```python
from build123d import *

# Parameters (mm, degrees)
F0_R     = 5
F1_DEPTH = 3


with BuildPart() as f1:
    # F0 (on Right) → F1 (new body)
    with BuildSketch(Plane.YZ):
        with BuildLine():
            ThreePointArc((30, 15), (15.633379, 6.233241), (0, 0))
            Line((0, 0), (30, 0))
            Line((30, 0), (30, -23))
            ThreePointArc((30, -23), (37.5, -30.5), (45, -23))
            Line((45, -23), (45, 6.824179))
            ThreePointArc((45, 6.824179), (43.227486, 10.642992), (39.166667, 11.754245))
            ThreePointArc((39.166667, 11.754245), (34.162235, 12.187856), (30, 15))
        make_face()
        with Locations((37.5, -23)):
            Circle(F0_R, mode=Mode.SUBTRACT)
    extrude(amount=F1_DEPTH)


solid = f1.part
```
The listing builds one solid part. Answer for the finished solid, in the listing's coordinates (mm). A direction names the side the tool comes from. Round coordinates to 2 decimals unless told otherwise and drop trailing zeros. Loops run counter-clockwise (first coordinate to the right, second up) from the corner with the lowest first, then second, coordinate; pieces in that order, holes last. Notation, with made-up numbers: (32.25, -6.5) - (47.25, -6.5) arc R15 cw to (47.25, 11.5) - close; hole circle Ø4 at (3, 14.25). An arc over 180 degrees is marked (long way). Use one line per item in the form item = value. Start each with the question number.
1. A tool of negligible diameter and unlimited length cuts with its end or side. For faces 1 (the face through (3, 32, -3)), 2 (the face through (1, 30, -11)), from which of +Z, -Z, +X, -X, +Y, -Y can it reach the whole face along a straight path? Write none if from no direction.
2. The part is cut by section C-C on z = -15. Determine the outline of the cut face in (x, y), then the cut area to 3 significant figures.
3. The part is cut by section A-A on y = 37.5. Determine the outline of the cut face in (x, z), then the cut area to 3 significant figures.
4. Consider line 1 (Z direction, x = 2.3, y = 37.5); line 2 (Y direction, x = 1.1, z = -20.5); line 3 (Y direction, x = 0.25, z = -21). Determine where each line is inside the solid, lowest interval first. Write a range as [from, to].
5. The part is cut by section B-B on x = 1.05. Determine the outline of the cut face in (y, z).
6. For a pull along Z with two mould halves and no side action, classify faces 3 (the face through (1, 15, 0)), 4 (the face through (1.5, 33.5, -26)), 5 (the face through (0, 32, -3)), 6 (the face through (1.479, 15.844, 6.339)) as pulls with the +Z half, pulls with the -Z half, needs draft (parallel to the pull), parting line crosses it, or undercut.
7. The part is cut by section D-D on y = 19.5. Determine the outline of the cut face in (x, z).
8. Given pin 1 Ø1.5 at (x, y) = (0.5, 14) entering from -Z, flat-ended and moving along its own axis, determine where the tip first touches the part or whether it passes through.
Geometry check:
q1.face_1 = +Z, -Z, +X, +Y, -Y
q1.face_2 = -Z, +X, -X, -Y
q2.outline = (0, 30) - (3, 30) - (3, 45) - (0, 45) - close
q2.area = 45.0 mm^2
q3.outline = (0, -30.5) - (3, -30.5) - (3, -28) - (0, -28) - close; (0, -18) - (3, -18) - (3, 11.61) - (0, 11.61) - close
q3.area = 96.3 mm^2
q4.line_1 = [-30.5, -28], [-18, 11.61]
q4.line_2 = [30, 33.17], [41.83, 45]
q4.line_3 = [30, 32.92], [42.08, 45]
q5.outline = (0, 0) - (30, 0) - (30, -23) arc R7.5 ccw to (45, -23) - (45, 6.82) arc R5 ccw to (39.17, 11.75) arc R10 cw to (30, 15) arc R100 cw to start; hole circle Ø10 at (37.5, -23)
q6.face_3 = pulls with the -Z half
q6.face_4 = undercut
q6.face_5 = needs draft
q6.face_6 = pulls with the +Z half
q7.outline = (0, 0) - (3, 0) - (3, 8.27) - (0, 8.27) - close
q8.pin_1 = 0
